Input: part model. Units: mm. Frame: model coordinates. Coordinates: 2 decimals unless noted, no trailing zeros. Loops run counter-clockwise (first coordinate to the right, second up) from the corner with the lowest first, then second, coordinate; pieces in that order, holes last.
Item 1: Ray query, line 1 along Y through (x, z) = (-51, 0.1); line 2 along Y through (x, z) = (59.5, 1.95); line 3 along X through (y, z) = (70, 1.9). Return the intervals inside material, ascending.
Item 2: Section A-A on x = -52.5. Return loops of the section in (y, z), and give its area (3 significant figures).
Item 3: Pull-direction query (X, two-part tool) for faces 1 (the cylindrical face through (141.846, 111.513, 0.986)), 2 (the flat face through (141.66, 57.99, 0.99)), 3 (the cylindrical face through (-148.21, 126.26, 0.99)); classes: released by +X, released by -X, zero draft, split by the parting line, or undercut.
Item 4: Section B-B on z = 0.6. Give the number of separate pieces and of enclosed holes in the cut face, and give its area (3 significant figures).
Item 5: Section C-C on y = 41. Return loops of the section in (x, z), and give its area (3 significant figures).
Item 6: Contact query for flat-ended pins moving along their axis: P1, Ø1, axis at x = 87, y = 82.5, coming from the -Z side; P2, Ø1, axis at y = 24.5, z = 1.5, coming from the +X side; P3, Ø1, axis at y = 97, z = 1.5, coming from the -X side. Output: stop coordinate, or through.
```python
from build123d import *

# Parameters (mm, degrees)
SKETCH3_R           = 1.6
SKETCH3_R_2         = 11
SKETCH3_R_3         = 4
BOSS_EXTRUDE1_DEPTH = 2
CUT_EXTRUDE3_DEPTH  = 3
SKETCH7_R           = 1.6
CUT_EXTRUDE4_DEPTH  = 3


with BuildPart() as part:
    # Sketch3 → Boss-Extrude1 (new body)
    with BuildSketch(Plane.XY):
        with BuildLine():
            ThreePointArc((-151.456383586, 112.587537538), (-148.084116861, 126.418210974), (-135.227817714, 132.531743734))
            Line((-135.227817714, 132.531743734), (133.810342842, 132.531743734))
            ThreePointArc((133.810342842, 132.531743734), (146.883625567, 126.475757693), (150.718078468, 112.587537538))
            Line((150.718078468, 112.587537538), (132.342869895, 1.839758932))
            ThreePointArc((132.342869895, 1.839758932), (120.43275171, -19.155269629), (97.771410342, -27.468256266))
            Line((97.771410342, -27.468256266), (-100, -27.468256266))
            ThreePointArc((-100, -27.468256266), (-117.356688592, -21.298876537), (-126.925740619, -5.558827984))
            Line((-126.925740619, -5.558827984), (-151.456383586, 112.587537538))
        make_face()
        with Locations((-114, 0.031743734)):
            Circle(SKETCH3_R, mode=Mode.SUBTRACT)
        with Locations((-100, -13.968256266)):
            Circle(SKETCH3_R, mode=Mode.SUBTRACT)
        with Locations((-86, 0.031743734)):
            Circle(SKETCH3_R, mode=Mode.SUBTRACT)
        with Locations((-100, 14.031743734)):
            Circle(SKETCH3_R, mode=Mode.SUBTRACT)
        with Locations((12.357913989, 16.531743734)):
            Circle(SKETCH3_R, mode=Mode.SUBTRACT)
        with Locations((12.357913989, 4.531743734)):
            Circle(SKETCH3_R, mode=Mode.SUBTRACT)
        with Locations((63.65613527, 10.531743734)):
            Circle(SKETCH3_R, mode=Mode.SUBTRACT)
        with Locations((-100, 0.031743734)):
            Circle(SKETCH3_R_2, mode=Mode.SUBTRACT)
        with Locations((100, 5.031743734)):
            Circle(SKETCH3_R_3, mode=Mode.SUBTRACT)
        with Locations((140, 115.061965544)):
            Circle(SKETCH3_R_3, mode=Mode.SUBTRACT)
        with Locations((-140, 115.061965544)):
            Circle(SKETCH3_R_3, mode=Mode.SUBTRACT)
        with BuildLine():
            ThreePointArc((-4, 108.133762314), (0, 104.133762314), (4, 108.133762314))
            Line((4, 108.133762314), (4, 121.990168775))
            ThreePointArc((4, 121.990168775), (0, 125.990168775), (-4, 121.990168775))
            Line((-4, 121.990168775), (-4, 108.133762314))
        make_face(mode=Mode.SUBTRACT)
    extrude(amount=BOSS_EXTRUDE1_DEPTH)

    # Sketch6 → Cut-Extrude3 (cut, through all)
    with BuildSketch(Plane.XY):
        with BuildLine():
            Line((-57.58, -17.298256266), (-37.58, -17.298256266))
            ThreePointArc((-37.58, -17.298256266), (-35.98, -18.898256266), (-37.58, -20.498256266))
            Line((-37.58, -20.498256266), (-57.58, -20.498256266))
            ThreePointArc((-57.58, -20.498256266), (-59.18, -18.898256266), (-57.58, -17.298256266))
        make_face()
        with BuildLine():
            Line((32.42, -17.298256266), (52.42, -17.298256266))
            ThreePointArc((52.42, -17.298256266), (54.02, -18.898256266), (52.42, -20.498256266))
            Line((52.42, -20.498256266), (32.42, -20.498256266))
            ThreePointArc((32.42, -20.498256266), (30.82, -18.898256266), (32.42, -17.298256266))
        make_face()
        with BuildLine():
            Line((-57.58, 125.561743734), (-37.58, 125.561743734))
            ThreePointArc((-37.58, 125.561743734), (-35.98, 123.961743734), (-37.58, 122.361743734))
            Line((-37.58, 122.361743734), (-57.58, 122.361743734))
            ThreePointArc((-57.58, 122.361743734), (-59.18, 123.961743734), (-57.58, 125.561743734))
        make_face()
        with BuildLine():
            Line((42.42, 125.561743734), (62.42, 125.561743734))
            ThreePointArc((62.42, 125.561743734), (64.02, 123.961743734), (62.42, 122.361743734))
            Line((62.42, 122.361743734), (42.42, 122.361743734))
            ThreePointArc((42.42, 122.361743734), (40.82, 123.961743734), (42.42, 125.561743734))
        make_face()
    extrude(amount=CUT_EXTRUDE3_DEPTH, mode=Mode.SUBTRACT)

    # Sketch7 → Cut-Extrude4 (cut, through all)
    with BuildSketch(Plane.XY.offset(2)):
        with Locations((-110.862196782, 95.074335332)):
            Circle(SKETCH7_R)
        with Locations((-73.908131188, 95.074335332)):
            Circle(SKETCH7_R)
        with Locations((-36.954065594, 95.074335332)):
            Circle(SKETCH7_R)
        with Locations((0, 95.074335332)):
            Circle(SKETCH7_R)
        with Locations((36.954065594, 95.074335332)):
            Circle(SKETCH7_R)
        with Locations((73.908131188, 95.074335332)):
            Circle(SKETCH7_R)
        with Locations((110.862196782, 95.074335332)):
            Circle(SKETCH7_R)
        with Locations((-73.908131188, 58.074335332)):
            Circle(SKETCH7_R)
        with Locations((-36.954065594, 58.074335332)):
            Circle(SKETCH7_R)
        with Locations((0, 58.074335332)):
            Circle(SKETCH7_R)
        with Locations((36.954065594, 58.074335332)):
            Circle(SKETCH7_R)
        with Locations((73.908131188, 58.074335332)):
            Circle(SKETCH7_R)
        with Locations((110.862196782, 58.074335332)):
            Circle(SKETCH7_R)
        with Locations((-73.908131188, 21.074335332)):
            Circle(SKETCH7_R)
        with Locations((-36.954065594, 21.074335332)):
            Circle(SKETCH7_R)
        with Locations((0, 21.074335332)):
            Circle(SKETCH7_R)
        with Locations((36.954065594, 21.074335332)):
            Circle(SKETCH7_R)
        with Locations((73.908131188, 21.074335332)):
            Circle(SKETCH7_R)
        with Locations((110.862196782, 21.074335332)):
            Circle(SKETCH7_R)
        with Locations((-110.862196782, 58.074335332)):
            Circle(SKETCH7_R)
        with Locations((-110.862196782, 21.074335332)):
            Circle(SKETCH7_R)
        with Locations((-141.184392471, 102.466753609)):
            Circle(SKETCH7_R)
        with Locations((-137.728402681, 85.821750317)):
            Circle(SKETCH7_R)
        with Locations((-134.272412891, 69.176747026)):
            Circle(SKETCH7_R)
        with Locations((-130.816423102, 52.531743734)):
            Circle(SKETCH7_R)
        with Locations((-127.360433312, 35.886740443)):
            Circle(SKETCH7_R)
        with Locations((-123.904443522, 19.241737151)):
            Circle(SKETCH7_R)
        with Locations((140.992053056, 102.843917034)):
            Circle(SKETCH7_R)
        with Locations((138.209463976, 86.0731926)):
            Circle(SKETCH7_R)
        with Locations((135.426874896, 69.302468167)):
            Circle(SKETCH7_R)
        with Locations((132.644285816, 52.531743734)):
            Circle(SKETCH7_R)
        with Locations((129.861696736, 35.761019301)):
            Circle(SKETCH7_R)
        with Locations((127.079107656, 18.990294868)):
            Circle(SKETCH7_R)
    extrude(amount=-CUT_EXTRUDE4_DEPTH, mode=Mode.SUBTRACT)


solid = part.part
```
Results found:
1. line 1: y = -27.47 to -20.5, -17.3 to 122.36, 125.56 to 132.53
1. line 2: y = -27.47 to 122.36, 125.56 to 132.53
1. line 3: x = -142.61 to -135.64, -132.9 to 133.99, 136.87 to 143.65
2. outline: (-27.47, 0) - (-20.5, 0) - (-20.5, 2) - (-27.47, 2) - close; (-17.3, 0) - (122.36, 0) - (122.36, 2) - (-17.3, 2) - close; (125.56, 0) - (132.53, 0) - (132.53, 2) - (125.56, 2) - close
2. area: 307 mm2
3. face 1: undercut
3. face 2: released by +X
3. face 3: released by -X
4. separate pieces: 1
4. enclosed holes: 49
4. area: 43,000 mm2
5. outline: (-136.59, 0) - (138.84, 0) - (138.84, 2) - (-136.59, 2) - close
5. area: 551 mm2
6. P1: stops at z = 0
6. P2: stops at x = 136.19
6. P3: stops at x = -148.32
